from build123d import *

# Parameters (mm, degrees)
SKETCH1_W                     = 735.584
SKETCH1_H                     = 38.1
WOOD_BLOCK_DEPTH              = 15.875
SKETCH2_R                     = 7.9375
INNER_BORE_DEPTH              = 737.741098814
SKETCH3_R                     = 6.35
MOUTHPIECE_THROUGH_HOLE_DEPTH = 737.741098814
SKETCH5_R                     = 8.128
CUT_EXTRUDE3_DEPTH            = 5.5499
SKETCH4_OUTSIDE_W             = 187.448
SKETCH4_OUTSIDE_H             = 165.223
SKETCH4_OUTSIDE_R             = 14.2875
OUTER_DIAMETER_DEPTH          = 737.741098916


with BuildPart() as part:
    # Sketch1 → wood block (new body)
    with BuildSketch(Plane(origin=(0, 0, 0), x_dir=(1, 0, 0), z_dir=(0, 1, 0))):
        with Locations((367.792, 19.05)):
            Rectangle(SKETCH1_W, SKETCH1_H)
    extrude(amount=WOOD_BLOCK_DEPTH)

    # Sketch2 → inner bore (cut, through all)
    with BuildSketch(Plane(origin=(735.584, 0, 0), x_dir=(0, 0, -1), z_dir=(1, 0, 0))):
        with Locations((19.05, 15.875)):
            Circle(SKETCH2_R)
    extrude(amount=-INNER_BORE_DEPTH, mode=Mode.SUBTRACT)

    # Sketch3 → mouthpiece through hole (cut, through all)
    with BuildSketch(Plane(origin=(0, 0, 0), x_dir=(1, 0, 0), z_dir=(0, 1, 0))):
        with Locations(Location((22.225, 19.05, 0), (0, 0, 90))):
            Circle(SKETCH3_R)
    extrude(amount=MOUTHPIECE_THROUGH_HOLE_DEPTH, mode=Mode.SUBTRACT)

    # Sketch5 → Cut-Extrude3 (cut)
    with BuildSketch(Plane.XZ):
        with Locations(Location((22.225, -19.05, 0), (0, 0, 270))):
            Circle(SKETCH5_R)
    extrude(amount=-CUT_EXTRUDE3_DEPTH, mode=Mode.SUBTRACT)

    # Sketch4 outside → outer diameter (cut, through all)
    with BuildSketch(Plane.ZY):
        with Locations((-19.05, 7.9375)):
            Rectangle(SKETCH4_OUTSIDE_W, SKETCH4_OUTSIDE_H)
        with Locations((-19.05, 15.875)):
            Circle(SKETCH4_OUTSIDE_R, mode=Mode.SUBTRACT)
    extrude(amount=-OUTER_DIAMETER_DEPTH, mode=Mode.SUBTRACT)


solid = part.part
Can you work these out from the model? Positions are in its coordinate system, mm. A direction names the side the tool comes from. Coordinates: 2 decimals unless noted, no trailing zeros. Loops run counter-clockwise (first coordinate to the right, second up) from the corner with the lowest first, then second, coordinate; pieces in that order, holes last. Notation, with made-up numbers: (33, -17.5) - (60, -17.5) arc R9 cw to (60, -8.5) - close; hole circle Ø7 at (36, 80.25). An arc over 180 degrees is marked (long way). Put each result on its own line as item: value. Start each with the question number.
Item 1: Suppose I cut it at A-A (z = -21). Please give me the cut outline in (x, y), and give its area (3 significant figures).
Item 2: If I drill on line 1 along Z through (x, y) = (583, 14.5); line 2 along X through (y, z) = (3.8, -19.05); line 3 along Y through (x, z) = (87, -19.25), over which ranges is the centre line in solid material (lowest first)?
Item 3: Which directions (+Z, -Z, +X, -X, +Y, -Y) give clear straight access to the entire face, cutting with the end or side of a thin tool? Please do faces 5 (the face through (19.112, 3.981, -26.558)), 6 (the face through (0, 7, -19)).
Item 4: For pin 1 (2 mm diameter, centred on y = 10, z = -13.5, fed in from -X); pin 2 (5 mm diameter, centred on x = 24, z = -18.5, fed in from -Y); pin 3 (1 mm diameter, centred on x = 504.5, y = 12.5, fed in from +Z); pin 4 (13 mm diameter, centred on x = 22.225, z = -19.05, fed in from -Y), each with a flat end and sliding along its axis, tell me the tip position at first contact or that it passes through.
Item 5: If we mould it in two halves opening along Z, with no side actions, what happens to faces 1 (the face through (28.424, 7.674, -17.673)), 2 (the face through (735.584, 7, -19)), 3 (the face through (362.64, 1.59, -19.36)), 4 (the face through (372.94, 7.94, -18.88))? For each: +Z half, -Z half, draft (parallel to the pull), parting line (faces both ways), or undercut.
Here are the results:
1. outline: (0, 1.72) - (14.33, 1.72) - (14.33, 5.55) - (16.18, 5.55) - (16.18, 8.18) - (0, 8.18) - close; (28.27, 5.55) - (30.12, 5.55) - (30.12, 1.72) - (735.58, 1.72) - (735.58, 8.18) - (28.27, 8.18) - close
1. area: 4,660 mm²
2. line 1: -33.27 to -26.87, -11.23 to -4.83
2. line 2: 0 to 14.1, 30.35 to 735.58
2. line 3: 1.59 to 7.94
3. face 5: -Y
3. face 6: +Z, -Z, -X, +Y, -Y
4. pin 1: x = 0
4. pin 2: through
4. pin 3: z = -5.05
4. pin 4: y = 5.55
5. face 1: undercut
5. face 2: draft
5. face 3: parting line
5. face 4: undercut
